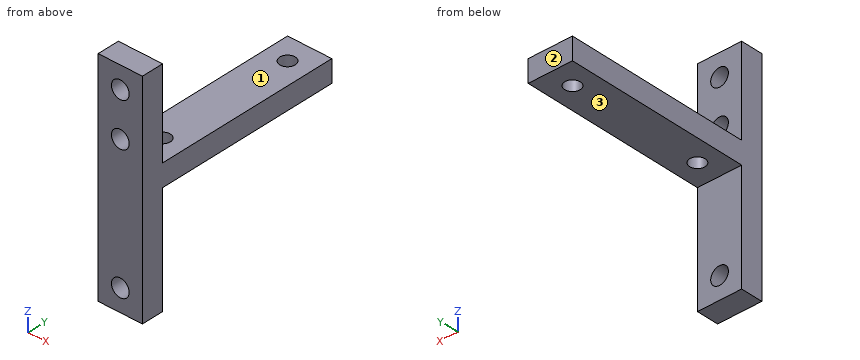
```python
from build123d import *

# Parameters (mm, degrees)
ESBO_O1_W                = 10
ESBO_O1_H                = 42
ESBO_O1_R                = 1.75
RESSALTO_EXTRUS_O1_DEPTH = 5
ESBO_O2_W                = 10
ESBO_O2_H                = 50
ESBO_O2_R                = 2
RESSALTO_EXTRUS_O2_DEPTH = 5


with BuildPart() as part:
    # Esboço1 → Ressalto-extrusão1 (new body)
    with BuildSketch(Plane.XY):
        Rectangle(ESBO_O1_W, ESBO_O1_H)
        with Locations((0, 15.5)):
            Circle(ESBO_O1_R, mode=Mode.SUBTRACT)
        with Locations((0, -15.5)):
            Circle(ESBO_O1_R, mode=Mode.SUBTRACT)
    extrude(amount=RESSALTO_EXTRUS_O1_DEPTH)

    # Esboço2 → Ressalto-extrusão2 (add)
    with BuildSketch(Plane.XZ.offset(21)):
        Rectangle(ESBO_O2_W, ESBO_O2_H)
        with Locations(Location((0, 20, 0), (0, 0, 270))):
            Circle(ESBO_O2_R, mode=Mode.SUBTRACT)
        with Locations(Location((0, -20, 0), (0, 0, 270))):
            Circle(ESBO_O2_R, mode=Mode.SUBTRACT)
        with Locations(Location((0, 10, 0), (0, 0, 270))):
            Circle(ESBO_O2_R, mode=Mode.SUBTRACT)
    extrude(amount=RESSALTO_EXTRUS_O2_DEPTH)


solid = part.part
```
Geometry check sheet. Reference: the model listing, model coordinates, mm. Face numbers are marked on the shaded views. A direction names the side the tool comes from. Round coordinates to 2 decimals unless told otherwise and drop trailing zeros. Order: outer loops, then holes, each group sorted by start corner. A loop starts at its lowest first (then second) coordinate and runs counter-clockwise, first axis right, second up. Notation, with made-up numbers: (59.5, -23.5) - (108.5, -23.5) arc R15 ccw to (108.5, 4.5) - close; hole circle Ø11 at (0.25, 29.5). An arc over 180 degrees is marked (long way). Use a Markdown table: item, result. Add a question column.
1) Set-up check for the marked faces 1, 2 and 3: record each of +Z, -Z, +X, -X, +Y, -Y from which the full face is reachable in a straight line by a thin tool's end or side.
2) Gauge pin test, flat ends, axial feed: P1, Ø4.5, axis at x = 0, y = -15.5, coming from the +Z side; P2, Ø5, axis at x = -2, z = -15, coming from the +Y side; P3, Ø1.5, axis at x = 0.5, y = -12.5, coming from the -Z side. Record the tip position at first contact, or that the pin passes through.
3) Thickness scan on line 1 along Y through (x, z) = (0, 1.5); line 2 along X through (y, z) = (-24.1, 10); line 3 along Z through (x, y) = (-4.25, 5). Record the ranges inside material, lowest first.
4) Section check C-C (x = 0). Record the cut outline in (y, z).
5) Section check A-A (z = 20). Record the cut outline in (x, y), then the cut area to 3 significant figures.
6) Section check B-B (y = 15.5). Record the cut outline in (x, z), then the cut area to 3 significant figures.
7) Section check D-D (x = -2.75). Record the cut outline in (y, z).
Established:
| question | item | result |
|---|---|---|
| 1 | face 1 | +Z, +X, -X, +Y |
| 1 | face 2 | +Z, -Z, +X, -X, +Y |
| 1 | face 3 | -Z, +X, -X, +Y |
| 2 | P1 | z = 5 |
| 2 | P2 | y = -21 |
| 2 | P3 | z = 0 |
| 3 | line 1 | -26 to -17.25, -13.75 to 13.75, 17.25 to 21 |
| 3 | line 2 | -5 to -2, 2 to 5 |
| 3 | line 3 | 0 to 5 |
| 4 | outline | (-26, -25) - (-21, -25) - (-21, -22) - (-26, -22) - close; (-26, -18) - (-21, -18) - (-21, 0) - (-17.25, 0) - (-17.25, 5) - (-21, 5) - (-21, 8) - (-26, 8) - close; (-26, 12) - (-21, 12) - (-21, 18) - (-26, 18) - close; (-26, 22) - (-21, 22) - (-21, 25) - (-26, 25) - close; (-13.75, 0) - (13.75, 0) - (13.75, 5) - (-13.75, 5) - close; (17.25, 0) - (21, 0) - (21, 5) - (17.25, 5) - close |
| 5 | outline | (-5, -26) - (-2, -26) - (-2, -21) - (-5, -21) - close; (2, -26) - (5, -26) - (5, -21) - (2, -21) - close |
| 5 | area | 30.0 mm2 |
| 6 | outline | (-5, 0) - (-1.75, 0) - (-1.75, 5) - (-5, 5) - close; (1.75, 0) - (5, 0) - (5, 5) - (1.75, 5) - close |
| 6 | area | 32.5 mm2 |
| 7 | outline | (-26, -25) - (-21, -25) - (-21, 0) - (21, 0) - (21, 5) - (-21, 5) - (-21, 25) - (-26, 25) - close |
